Input: dimensioned drawing with shaded views. Units: mm. Origin: part minimum x, y, z. Give positions to 0.01 mm unless a question says otherwise; leave off trailing zeros. Write each loop counter-clockwise with the first axis right and the second up, starting at its lowest first coordinate (ties: lowest second). Pieces come first, ordered by that corner, then holes. Notation, with made-up numbers: (13.25, 0) - (17.25, 0) arc R23 ccw to (17.25, 35) - close; hole circle Ø5 at (29, 23). An arc over 180 degrees is marked (long way). Answer as a JSON object with one key per item and string values. Group by question number.
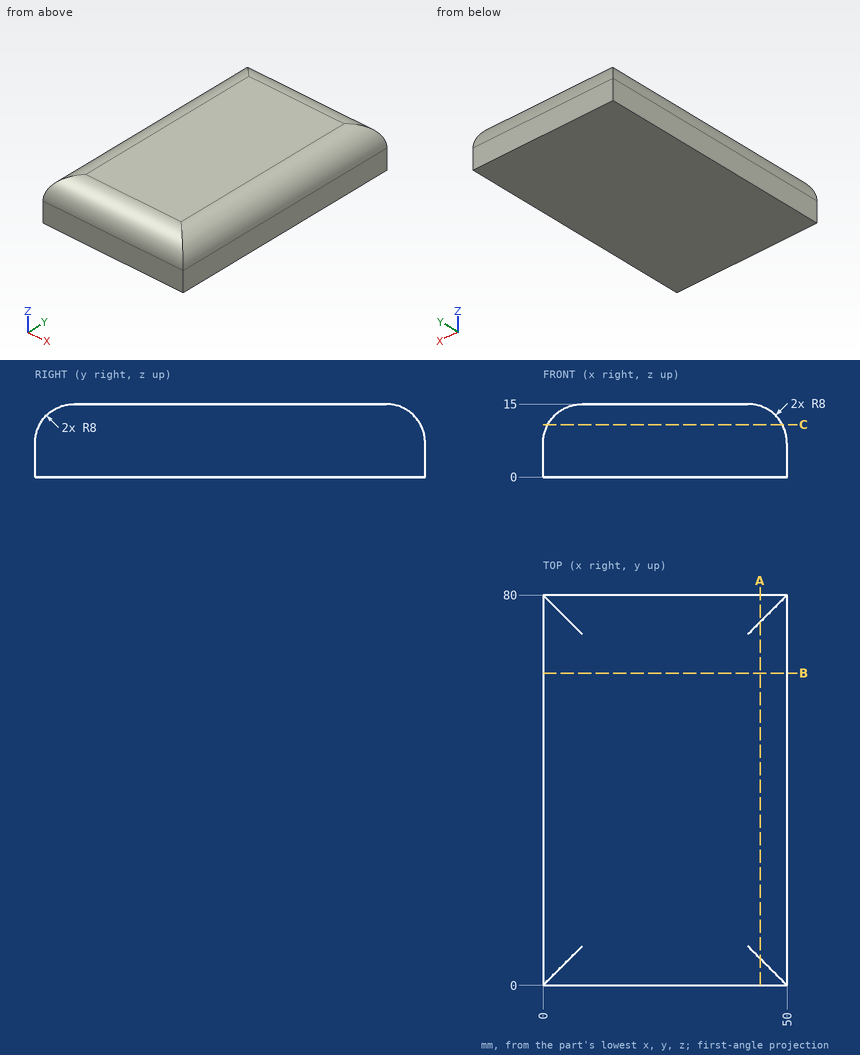
Q1. Section C-C on z = 10.75. Return the cut outline in (x, y), then the cut area to 3 significant figures.
Q2. Section A-A on x = 44.5. Return the cut outline in (y, z).
Q3. First-contact query: pin 1 Ø6 at (y, z) = (62, 10.5) entering from -X; pin 2 Ø1.5 at (x, z) = (44, 10) entering from -Y. Flat tips, straight axial feed; report the tip coordinate or a pass-through.
Q4. Section B-B on y = 64. Return the cut outline in (x, z).
Q5. Ray query, probe 1 along Y at (x, z) = (39, 13.75); probe 2 along X at (y, z) = (3, 11.5); probe 3 along X at (y, z) = (56, 7.25). Return the intervals inside material, ascending. Write a range as [from, to].
Taken from the geometry:
{
 "1": {"outline": "(0.93, 0.93) - (49.07, 0.93) - (49.07, 79.07) - (0.93, 79.07) - close", "area": "3,760 mm²"},
 "2": {"outline": "(0, 0) - (80, 0) - (80, 7) arc R8 ccw to (74.5, 14.6) - (5.5, 14.6) arc R8 ccw to (0, 7) - close"},
 "3": {"pin 1": "stops at x = 0.02", "pin 2": "stops at y = 0.32"},
 "4": {"outline": "(0, 0) - (50, 0) - (50, 7) arc R8 ccw to (42, 15) - (8, 15) arc R8 ccw to (0, 7) - close"},
 "5": {"probe 1": "y = [3.71, 76.29]", "probe 2": "x = [1.39, 48.61]", "probe 3": "x = [0, 50]"}
}
